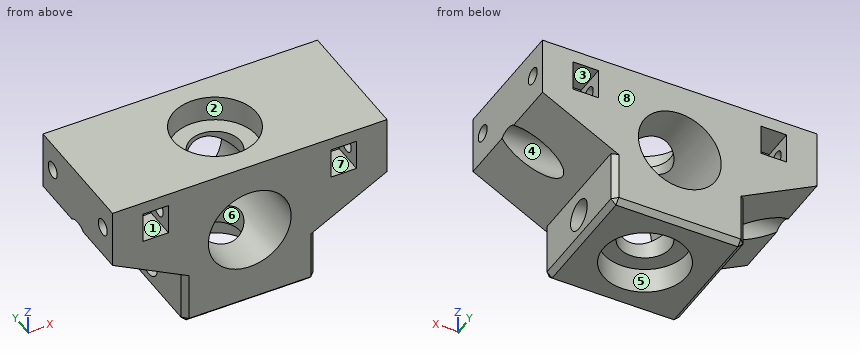
from build123d import *

# Parameters (mm, degrees)
SKETCH1_R               = 8.15
BOSS_EXTRUDE1_DEPTH     = 25
SKETCH2_R               = 5
CUT_EXTRUDE1_DEPTH      = 48.476309882
SKETCH3_R               = 8.2
CUT_EXTRUDE2_DEPTH      = 5
CUT_EXTRUDE3_START      = -5
SKETCH4_R               = 8.2
CUT_EXTRUDE3_DEPTH      = 5
CHAMFER1_SIZE           = 1
CUT_EXTRUDE4_DEPTH      = 41.124805358
CUT_EXTRUDE4_DEPTH_BACK = 41.124805358
SKETCH5_R               = 1.25
CUT_EXTRUDE5_START      = -13
SKETCH6_R               = 3.25
CUT_EXTRUDE5_DEPTH      = 28.124805358
SKETCH7_R               = 3
CUT_EXTRUDE6_DEPTH      = 4
SKETCH9_R               = 1.6
CUT_EXTRUDE7_DEPTH      = 14
CUT_EXTRUDE8_START      = -6
CUT_EXTRUDE8_DEPTH      = 5


with BuildPart() as part:
    # Sketch1 → Boss-Extrude1 (new body)
    with BuildSketch(Plane(origin=(0, 0, 0), x_dir=(1, 0, 0), z_dir=(0, 1, 0))):
        Polygon((-13, 14), (-13, 5), (-27, -2.5), (-27, -14), (27, -14), (27, -2.5), (13, 5), (13, 14), (13, 16), (-13, 16), align=None)
        with Locations(Location((0, 0, 0), (0, 0, 270))):
            Circle(SKETCH1_R, mode=Mode.SUBTRACT)
    extrude(amount=BOSS_EXTRUDE1_DEPTH)

    # Sketch2 → Cut-Extrude1 (cut, through all)
    with BuildSketch(Plane.XY.offset(14)):
        with Locations((0, 12.5)):
            Circle(SKETCH2_R)
    extrude(amount=-CUT_EXTRUDE1_DEPTH, mode=Mode.SUBTRACT)

    # Sketch3 → Cut-Extrude2 (cut)
    with BuildSketch(Plane(origin=(0, 0, -16), x_dir=(-1, 0, 0), z_dir=(0, 0, -1))):
        with Locations((0, 12.5)):
            Circle(SKETCH3_R)
    extrude(amount=-CUT_EXTRUDE2_DEPTH, mode=Mode.SUBTRACT)

    # Sketch4 → Cut-Extrude3 (cut)
    with BuildSketch(Plane.XY.offset(14).offset(CUT_EXTRUDE3_START)):
        with Locations(Location((0, 12.5, 0), (0, 0, 180))):
            Circle(SKETCH4_R)
    extrude(amount=CUT_EXTRUDE3_DEPTH, mode=Mode.SUBTRACT)

    # Chamfer1
    chamfer1_edges = [part.edges().sort_by_distance(p)[0] for p in [
        (-13, 0, -10.5),
        (-13, 12.5, -16),
        (13, 12.5, -16),
        (13, 25, -10.5),
        (0, 25, -16),
        (-13, 25, -10.5),
        (0, 0, -16),
        (13, 0, -10.5),
    ]]
    chamfer(chamfer1_edges, length=CHAMFER1_SIZE)

    # Sketch5 → Cut-Extrude4 (cut, two sides: drawn at the far end of the back side and taken through both)
    with BuildSketch(Plane(origin=(0, 0, 0), x_dir=(0, 0, -1), z_dir=(1, 0, 0)).offset(-CUT_EXTRUDE4_DEPTH_BACK)):
        with Locations((0, 12.546077806)):
            Circle(SKETCH5_R)
    extrude(amount=CUT_EXTRUDE4_DEPTH + CUT_EXTRUDE4_DEPTH_BACK, mode=Mode.SUBTRACT)

    # Sketch6 → Cut-Extrude5 (cut, through all)
    with BuildSketch(Plane(origin=(0, 0, 0), x_dir=(0, 0, -1), z_dir=(1, 0, 0)).offset(CUT_EXTRUDE5_START)):
        with Locations((0, 12.546077806)):
            Circle(SKETCH6_R)
    cut_extrude5 = extrude(amount=-CUT_EXTRUDE5_DEPTH, mode=Mode.SUBTRACT)

    # Mirror1: Cut-Extrude5 across plane
    add(cut_extrude5.mirror(Plane(origin=(0, 0, 0), x_dir=(0, 0, 1), z_dir=(1, 0, 0))), mode=Mode.SUBTRACT)

    # Sketch7 → Cut-Extrude6 (cut)
    with BuildSketch(Plane(origin=(13, 0, 0), x_dir=(0, 0, -1), z_dir=(1, 0, 0))):
        with Locations((10.5, 12.5)):
            Circle(SKETCH7_R)
    cut_extrude6 = extrude(amount=-CUT_EXTRUDE6_DEPTH, mode=Mode.SUBTRACT)

    # Sketch9 → Cut-Extrude7 (cut)
    with BuildSketch(Plane(origin=(27, 0, 0), x_dir=(0, 0, -1), z_dir=(1, 0, 0))):
        with Locations((-8.5, 21.5)):
            Circle(SKETCH9_R)
        with Locations((-8.5, 3.5)):
            Circle(SKETCH9_R)
    cut_extrude7 = extrude(amount=-CUT_EXTRUDE7_DEPTH, mode=Mode.SUBTRACT)

    # Sketch10 → Cut-Extrude8 (cut)
    with BuildSketch(Plane(origin=(27, 0, 0), x_dir=(0, 0, -1), z_dir=(1, 0, 0)).offset(CUT_EXTRUDE8_START)):
        Polygon((-11.5, 19.767949192), (-11.5, 18.767949192), (-8.5, 17.035898385), (-5.5, 18.767949192), (-5.5, 19.767949192), (-5.5, 23.232050808), (-5.5, 25), (-11.5, 25), (-11.5, 23.232050808), align=None)
        Polygon((-11.5, 0), (-11.5, 1.767949192), (-11.5, 5.232050808), (-11.5, 6.232050808), (-8.5, 7.964101615), (-5.5, 6.232050808), (-5.5, 5.232050808), (-5.5, 1.767949192), (-5.5, 0), align=None)
    cut_extrude8 = extrude(amount=-CUT_EXTRUDE8_DEPTH, mode=Mode.SUBTRACT)

    # Mirror2: Cut-Extrude6, Cut-Extrude7, Cut-Extrude8 across plane
    add(cut_extrude6.mirror(Plane(origin=(0, 0, 0), x_dir=(0, 0, 1), z_dir=(1, 0, 0))), mode=Mode.SUBTRACT)
    add(cut_extrude7.mirror(Plane(origin=(0, 0, 0), x_dir=(0, 0, 1), z_dir=(1, 0, 0))), mode=Mode.SUBTRACT)
    add(cut_extrude8.mirror(Plane(origin=(0, 0, 0), x_dir=(0, 0, 1), z_dir=(1, 0, 0))), mode=Mode.SUBTRACT)


solid = part.part
The listing builds one solid part. Answer for the finished solid, in the listing's coordinates (mm). Face numbers are marked on the shaded views. A direction names the side the tool comes from. Give positions to 0.01 mm unless a question says otherwise; leave off trailing zeros. Write each loop counter-clockwise with the first axis right and the second up, starting at its lowest first coordinate (ties: lowest second). Pieces come first, ordered by that corner, then holes. Notation, with made-up numbers: (60, -15) - (78, -15) arc R16 ccw to (78, 9) - close; hole circle Ø10 at (-35, 67.5). An arc over 180 degrees is marked (long way). Use a Markdown table: item, result.
1. Section A-A on x = 0 is taken. Write down the section's boundary in (y, z).
Values follow:
| item | result |
|---|---|
| outline | (0, -15) - (1, -16) - (4.3, -16) - (4.3, -11) - (7.5, -11) - (7.5, -8.15) - (0, -8.15) - close; (0, 8.15) - (7.5, 8.15) - (7.5, 9) - (4.3, 9) - (4.3, 14) - (0, 14) - close; (17.5, -11) - (20.7, -11) - (20.7, -16) - (24, -16) - (25, -15) - (25, -8.15) - (17.5, -8.15) - close; (17.5, 8.15) - (25, 8.15) - (25, 14) - (20.7, 14) - (20.7, 9) - (17.5, 9) - close |
2. Section C-C on x = -22.5 is taken. Write down the section's boundary in (y, z).
Values follow:
| item | result |
|---|---|
| outline | (0, 0.09) - (9.3, 0.09) arc R3.25 cw to (15.79, 0.09) - (25, 0.09) - (25, 14) - (0, 14) - close; hole circle Ø3.2 at (3.5, 8.5); hole circle Ø3.2 at (21.5, 8.5) |
3. Section D-D on z = -0.25 is taken. Write down the section's boundary in (x, y).
Values follow:
| item | result |
|---|---|
| outline | (-21.87, 0) - (-8.15, 0) - (-8.15, 11.32) - (-13, 11.32) - (-13, 9.31) - (-21.87, 9.31) - close; (-21.87, 15.79) - (-13, 15.79) - (-13, 13.77) - (-8.15, 13.77) - (-8.15, 25) - (-21.87, 25) - close; (8.15, 0) - (21.87, 0) - (21.87, 9.31) - (13, 9.31) - (13, 11.32) - (8.15, 11.32) - close; (8.15, 13.77) - (13, 13.77) - (13, 15.79) - (21.87, 15.79) - (21.87, 25) - (8.15, 25) - close |
4. For a pull along Y with two mould halves and no side action, classify the marked faces 6, 7 and 8 as released by +Y, released by -Y, zero draft, split by the parting line, or undercut.
Values follow:
| item | result |
|---|---|
| face 6 | undercut |
| face 7 | zero draft |
| face 8 | released by +Y |
5. Section B-B on z = -4 is taken. Write down the section's boundary in (x, y).
Values follow:
| item | result |
|---|---|
| outline | (-14.87, 0) - (-7.1, 0) - (-7.1, 25) - (-14.87, 25) - close; (7.1, 0) - (14.87, 0) - (14.87, 25) - (7.1, 25) - close |
6. Each of these flat-tipped pins is pushed along its axis until it touches: P1, Ø12, axis at y = 15.5, z = -4, coming from the -X side; P2, Ø3, axis at y = 13, z = -1, coming from the +X side; P3, Ø4, axis at y = 17, z = -0.5, coming from the -X side; P4, Ø1.5, axis at y = 12.55, z = 0, coming from the +X side. Where does it stop, or does it pass through?
Values follow:
| item | result |
|---|---|
| P1 | stops at x = -26.07 |
| P2 | stops at x = 13 |
| P3 | stops at x = -25.13 |
| P4 | passes through |
7. A tool of negligible diameter and unlimited length cuts with its end or side. For the marked faces 1, 2, 3, 4 and 5, from which of +Z, -Z, +X, -X, +Y, -Y can it reach the whole face along a straight path? Write none if from no direction.
Values follow:
| item | result |
|---|---|
| face 1 | -Y |
| face 2 | +Z |
| face 3 | +Y |
| face 4 | +X |
| face 5 | -Z |
8. Find the intervals of material crossed by probe 1 along Y at (x, z) = (-25.35, 8.5); probe 2 along Y at (x, z) = (11.1, 0); probe 3 along Y at (x, z) = (-24, 8), in increasing order. Write a range as from..to.
Values follow:
| item | result |
|---|---|
| probe 1 | y = 0..1.9, 5.1..19.9, 23.1..25 |
| probe 2 | y = 0..11.3, 13.8..25 |
| probe 3 | y = 0..1.98, 5.02..19.98, 23.02..25 |
